Geometry check sheet. Reference: the model listing, model coordinates, mm. Face numbers are marked on the shaded views. A direction names the side the tool comes from. Round coordinates to 2 decimals unless told otherwise and drop trailing zeros. Write each loop counter-clockwise with the first axis right and the second up, starting at its lowest first coordinate (ties: lowest second). Pieces come first, ordered by that corner, then holes.
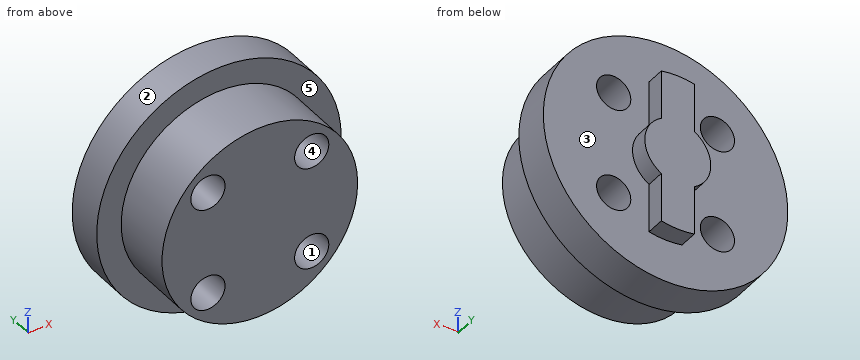
from build123d import *

# Parameters (mm, degrees)
SKETCH1_R           = 10
BOSS_EXTRUDE1_DEPTH = 8
BOSS_EXTRUDE2_DEPTH = 1.5
SKETCH5_R           = 10
SKETCH5_R_2         = 8
CUT_EXTRUDE1_DEPTH  = 5
SKETCH6_R           = 1.4
CUT_EXTRUDE2_DEPTH  = 8
CIRPATTERN1_COUNT   = 4


with BuildPart() as part:
    # Sketch1 → Boss-Extrude1 (new body)
    with BuildSketch(Plane(origin=(0, 0, 0), x_dir=(1, 0, 0), z_dir=(0, 1, 0))):
        Circle(SKETCH1_R)
    extrude(amount=BOSS_EXTRUDE1_DEPTH)

    # Sketch4 → Boss-Extrude2 (add)
    with BuildSketch(Plane(origin=(0, 8, 0), x_dir=(1, 0, 0), z_dir=(0, 1, 0))):
        with BuildLine():
            Line((-1.35, 6.358262341), (-1.35, 2.33826859))
            ThreePointArc((-1.35, 2.33826859), (-2.7, 0), (-1.35, -2.33826859))
            Line((-1.35, -2.33826859), (-1.35, -6.358262341))
            ThreePointArc((-1.35, -6.358262341), (0, -6.5), (1.35, -6.358262341))
            Line((1.35, -6.358262341), (1.35, -2.33826859))
            ThreePointArc((1.35, -2.33826859), (2.7, 0), (1.35, 2.33826859))
            Line((1.35, 2.33826859), (1.35, 6.358262341))
            ThreePointArc((1.35, 6.358262341), (0, 6.5), (-1.35, 6.358262341))
        make_face()
    extrude(amount=BOSS_EXTRUDE2_DEPTH)

    # Sketch5 → Cut-Extrude1 (cut)
    with BuildSketch(Plane(origin=(0, 0, 0), x_dir=(1, 0, 0), z_dir=(0, 1, 0))):
        Circle(SKETCH5_R)
        Circle(SKETCH5_R_2, mode=Mode.SUBTRACT)
    extrude(amount=CUT_EXTRUDE1_DEPTH, mode=Mode.SUBTRACT)

    # Sketch6 → Cut-Extrude2 (cut)
    with BuildSketch(Plane.XZ):
        with Locations((4.242640687, 4.242640687)):
            Circle(SKETCH6_R)
    cut_extrude2 = extrude(amount=-CUT_EXTRUDE2_DEPTH, mode=Mode.SUBTRACT)

    # CirPattern1: Cut-Extrude2 ×4 about axis
    cirpattern1_axis = Axis((0, 0, 0), (0, 1, 0))
    for i in range(1, CIRPATTERN1_COUNT):
        add(cut_extrude2.rotate(cirpattern1_axis, i * 360 / CIRPATTERN1_COUNT), mode=Mode.SUBTRACT)


solid = part.part
1. Section check C-C (x = 0). Record the cut outline in (y, z), plus the area to 4 significant figures.
2. Section check A-A (z = -3.75). Record the cut outline in (x, y).
3. Section check D-D (z = 0). Record the cut outline in (x, y).
4. Scan lines: line 1 along X through (y, z) = (5.5, 3.25); line 2 along X through (y, z) = (5.5, 3.5); line 3 along Z through (x, y) = (-5, 4.25) (3 decimals). Record each from-to range of solid material in increasing order.
5. Depth check by flat-ended pin: pin 1 Ø3 at (x, z) = (-4.24, -4.24) entering from +Y; pin 2 Ø0.8 at (y, z) = (9, 4.5) entering from -X; pin 3 Ø1.6 at (y, z) = (8.5, -4) entering from +X. Enter the tip coordinate at first touch or a pass-through.
6. Release check for a two-part mould opening along X. For the marked faces 1, 2 and 3 record: +X half, -X half, draft (parallel to the pull), parting line (faces both ways), or undercut.
7. Section check B-B (y = 8.5). Record the cut outline in (x, z).
8. Access from +Z, -Z, +X, -X, +Y, -Y to the whole of each face (thin tool, end or side, straight path). Record for the marked faces 4 and 5.
Results below:
1. outline: (0, -8) - (5, -8) - (5, -10) - (8, -10) - (8, -6.5) - (9.5, -6.5) - (9.5, 6.5) - (8, 6.5) - (8, 10) - (5, 10) - (5, 8) - (0, 8) - close
1. area: 159.5 mm2
2. outline: (-9.27, 5) - (-7.07, 5) - (-7.07, 0) - (-5.55, 0) - (-5.55, 8) - (-9.27, 8) - close; (-2.93, 0) - (2.93, 0) - (2.93, 8) - (1.35, 8) - (1.35, 9.5) - (-1.35, 9.5) - (-1.35, 8) - (-2.93, 8) - close; (5.55, 0) - (7.07, 0) - (7.07, 5) - (9.27, 5) - (9.27, 8) - (5.55, 8) - close
3. outline: (-10, 5) - (-8, 5) - (-8, 0) - (8, 0) - (8, 5) - (10, 5) - (10, 8) - (2.7, 8) - (2.7, 9.5) - (-2.7, 9.5) - (-2.7, 8) - (-10, 8) - close
4. line 1: x = -9.46 to -5.23, -3.26 to 3.26, 5.23 to 9.46
4. line 2: x = -9.37 to -5.43, -3.06 to 3.06, 5.43 to 9.37
4. line 3: z = -6.245 to -5.42, -3.065 to 3.065, 5.42 to 6.245
5. pin 1: stops at y = 8
5. pin 2: stops at x = -1.35
5. pin 3: stops at x = 9.41
6. face 1: undercut
6. face 2: parting line
6. face 3: draft
7. outline: (-1.35, -6.36) arc R6.5 ccw to (1.35, -6.36) - (1.35, -2.34) arc R2.7 ccw to (1.35, 2.34) - (1.35, 6.36) arc R6.5 ccw to (-1.35, 6.36) - (-1.35, 2.34) arc R2.7 ccw to (-1.35, -2.34) - close
8. face 4: +Y, -Y
8. face 5: -Y
